The listing builds one solid part. Answer for the finished solid, in the listing's coordinates (mm). A direction names the side the tool comes from. Coordinates: 2 decimals unless noted, no trailing zeros. Order: outer loops, then holes, each group sorted by start corner. A loop starts at its lowest first (then second) coordinate and runs counter-clockwise, first axis right, second up. Notation, with made-up numbers: (63, 6.25) -> (101, 6.25) arc R36 cw to (101, 41.25) -> close; hole circle Ø9 at (35, 83.5). An arc over 180 degrees is marked (long way). Return JSON: item names as keys, results as strings.
from build123d import *

# Parameters (mm, degrees)
BOSS_EXTRUDE1_DEPTH     = 25.4
SHELL1_T                = -1.27
CUT_EXTRUDE1_DEPTH      = 32.894396236
CUT_EXTRUDE1_DEPTH_BACK = 32.894396236
SKETCH2_R               = 0.635
CUT_EXTRUDE3_DEPTH      = 7.874
CUT_EXTRUDE3_DEPTH_BACK = 7.874
SKETCH4_R               = 1.27
CUT_EXTRUDE2_DEPTH      = 0.762
CUT_EXTRUDE4_START      = -17.111468296
CUT_EXTRUDE4_OUTLINE_W  = 0.990065124
CUT_EXTRUDE4_OUTLINE_H  = 2.54
CUT_EXTRUDE4_DEPTH      = 0.508


# Read off the part's stored shape, not the designer's step: Cut-Extrude4
with BuildPart() as part:
    # Sketch1 → Boss-Extrude1 (new body)
    with BuildSketch(Plane(origin=(0, 0, 0), x_dir=(0, 0, -1), z_dir=(1, 0, 0))):
        with BuildLine():
            Line((-4.445, 0), (4.445, 0))
            Line((4.445, 0), (8.89, -7.69896584))
            ThreePointArc((8.89, -7.69896584), (0, -17.111468296), (-8.89, -7.69896584))
            Line((-8.89, -7.69896584), (-4.445, 0))
        make_face()
    extrude(amount=BOSS_EXTRUDE1_DEPTH)

    # Shell1
    shell1_openings = [part.faces().sort_by_distance(p)[0] for p in [
        (25.4, -8.481857982, 0),
        (0, -8.481857982, 0),
    ]]
    offset(amount=SHELL1_T, openings=shell1_openings, kind=Kind.INTERSECTION)

    # Sketch2 → Cut-Extrude1 (cut, two sides: drawn at the far end of the back side and taken through both)
    with BuildSketch(Plane.XY.offset(-CUT_EXTRUDE1_DEPTH_BACK)):
        with Locations((22.5978056, -7.69896584)):
            Circle(SKETCH2_R)
        with BuildLine():
            Line((25.4, 0), (23.032171182, -6.505556211))
            ThreePointArc((23.032171182, -6.505556211), (23.724309358, -8.285386578), (21.869363526, -8.739288936))
            Line((21.869363526, -8.739288936), (16.007100426, -17.111468296))
            Line((16.007100426, -17.111468296), (25.4, -17.111468296))
            Line((25.4, -17.111468296), (25.4, 0))
        make_face()
        Polygon((0, 0), (6.228065124, -17.111468296), (0, -17.111468296), align=None)
    extrude(amount=CUT_EXTRUDE1_DEPTH + CUT_EXTRUDE1_DEPTH_BACK, mode=Mode.SUBTRACT)

    # Sketch4 → Cut-Extrude3 (cut, two sides: drawn at the far end of the back side and taken through both)
    with BuildSketch(Plane.XY.offset(-CUT_EXTRUDE3_DEPTH_BACK)):
        with Locations((22.5978056, -7.69896584)):
            Circle(SKETCH4_R)
    extrude(amount=CUT_EXTRUDE3_DEPTH + CUT_EXTRUDE3_DEPTH_BACK, mode=Mode.SUBTRACT)

    # Sketch3 → Cut-Extrude2 (cut)
    with BuildSketch(Plane(origin=(0, 0, 0), x_dir=(1, 0, 0), z_dir=(0, 1, 0))):
        Polygon((3.621972553, 1.783922101), (3.906908451, 1.783922101), (3.906908451, 0.57485259), (5.230461135, 1.783922101), (5.6368764, 1.783922101), (4.076725158, 0.359242614), (5.758991784, -1.391077899), (5.37928926, -1.391077899), (3.906908451, 0.141088567), (3.906908451, -1.391077899), (3.621972553, -1.391077899), align=None)
        Polygon((6.227100758, 1.783922101), (6.512036656, 1.783922101), (6.512036656, -1.065436874), (7.733190502, -1.065436874), (7.733190502, -1.391077899), (6.227100758, -1.391077899), align=None)
        Polygon((8.058831528, 1.783922101), (8.35330769, 1.783922101), (8.974696912, -0.544538436), (9.898830526, 1.783922101), (9.940171672, 1.783922101), (10.84713281, -0.528637995), (11.471702121, 1.783922101), (11.762998194, 1.783922101), (10.906918467, -1.391077899), (10.866213339, -1.391077899), (9.910914861, 1.037237405), (8.944168066, -1.391077899), (8.903462938, -1.391077899), align=None)
        Polygon((12.170049476, 1.458281075), (12.170049476, 1.783922101), (13.838959733, 1.783922101), (12.507138819, -1.065436874), (13.798254605, -1.065436874), (13.798254605, -1.391077899), (12.047934092, -1.391077899), (13.379755005, 1.458281075), align=None)
    extrude(amount=-CUT_EXTRUDE2_DEPTH, mode=Mode.SUBTRACT)

    # Cut-Extrude4 outline → Cut-Extrude4 (cut)
    with BuildSketch(Plane(origin=(0, 0, 0), x_dir=(1, 0, 0), z_dir=(0, 1, 0)).offset(CUT_EXTRUDE4_START)):
        with Locations((6.495032562, 0)):
            Rectangle(CUT_EXTRUDE4_OUTLINE_W, CUT_EXTRUDE4_OUTLINE_H)
    extrude(amount=CUT_EXTRUDE4_DEPTH, mode=Mode.SUBTRACT)


solid = part.part
1. Each of these flat-tipped pins is pushed along its axis until it touches: pin 1 Ø0.6 at (y, z) = (-0.5, 0) entering from -X; pin 2 Ø0.8 at (x, y) = (13, -0.5) entering from -Z; pin 3 Ø1 at (x, y) = (15, -12) entering from +Z. Where does it stop, or does it pass through?
Answer block:
{"pin 1": "stops at x = 0.07", "pin 2": "stops at z = -4.96", "pin 3": "stops at z = 8.27"}
2. The part is cut by section D-D on x = 9.5. Give the vertices of the cut face in (y, z) (1 decimal).
Answer block:
{"outline": "(-7.7, -8.9) -> (0, -4.4) -> (0, -0.8) -> (-0.8, -0.8) -> (-0.8, 0) -> (0, 0) -> (0, 4.4) -> (-7.7, 8.9) arc R8.9 ccw (long way) to start; hole (-8.1, -7.6) -> (-1.3, -3.7) -> (-1.3, 3.7) -> (-8.1, 7.6) arc R7.6 ccw (long way) to start"}
3. Consider line 1 (Z direction, x = 12.75, y = -14); line 2 (Z direction, x = 19, y = -5.5); line 3 (Y direction, x = 21.25, z = 2.25). Determine where each line is inside the solid, lowest interval first. Write a range as from..to.
Answer block:
{"line 1": "z = -6.76..-4.97, 4.97..6.76", "line 2": "z = -7.62..-6.15, 6.15..7.62", "line 3": "y = -1.27..0"}
4. For faces 4 (the face through (23.45, -8.64, 8.38)), 5 (the face through (6.5, -16.603, 0)), 6 (the face through (21.7, -6.8, -7.4)), 7 (the face through (4.56, -0.38, -1.17)), determine the directions among +Z, -Z, +X, -X, +Y, -Y from which every point of the face is accessible in a straight line to the end or side of a thin tool.
Answer block:
{"face 4": "+Z, -Z", "face 5": "-X, -Y", "face 6": "none", "face 7": "+Y"}
5. The part is cut by section A-A on y = -4.25. Give the vertices of the cut face in (x, z).
Answer block:
{"outline": "(1.55, -6.9) -> (23.85, -6.9) -> (23.85, -5.43) -> (1.55, -5.43) -> close; (1.55, 5.43) -> (23.85, 5.43) -> (23.85, 6.9) -> (1.55, 6.9) -> close"}
6. The part is cut by section B-B on z = 4.75. Give the vertices of the cut face in (x, y).
Answer block:
{"outline": "(0.19, -0.53) -> (1.12, -3.07) -> (24.28, -3.07) -> (25.21, -0.53) -> close; (5.16, -14.18) -> (5.73, -15.74) -> (16.97, -15.74) -> (18.06, -14.18) -> close"}
7. Determine the mould class of faces 1 (the face through (16.78, -16.01, 0.62)), 2 (the face through (10.39, -0.38, -0.64)), 3 (the face through (10.85, -17.11, -0.2)) for opening direction Z: pulls with the +Z half, pulls with the -Z half, needs draft (parallel to the pull), parting line crosses it, or undercut.
Answer block:
{"face 1": "needs draft", "face 2": "undercut", "face 3": "parting line crosses it"}
8. The part is cut by section C-C on x = 22.5. Give the vertices of the cut face in (y, z) (1 decimal), and give its area (3 significant figures).
Answer block:
{"outline": "(-9, -8.9) arc R8.9 ccw to (-8.3, -8.9) -> (-8.3, -7.9) -> (-9, -7.9) -> close; (-9, 7.9) -> (-8.3, 7.9) -> (-8.3, 8.9) arc R8.9 ccw to (-9, 8.9) -> close; (-7.1, -8.5) -> (0, -4.4) -> (0, 4.4) -> (-7.1, 8.5) -> (-7.1, 7.9) -> (-6.4, 7.9) -> (-6.4, 6.7) -> (-1.3, 3.7) -> (-1.3, -3.7) -> (-6.4, -6.7) -> (-6.4, -7.9) -> (-7.1, -7.9) -> close", "area": "29.3 mm2"}
